```python
from build123d import *

# Parameters (mm, degrees)
BOSS_EXTRUDE1_DEPTH = 38.1
SKETCH2_R           = 17.78
CUT_EXTRUDE1_DEPTH  = 142.514046179


with BuildPart() as part:
    # Sketch1 → Boss-Extrude1 (new body, symmetric)
    with BuildSketch(Plane.XY):
        with BuildLine():
            Line((0, 0), (-177.8, 0))
            Line((-177.8, 0), (-454.042613489, -128.814046179))
            Line((-454.042613489, -128.814046179), (-459.409865413, -117.303937283))
            Line((-459.409865413, -117.303937283), (-183.167251924, 11.510108895))
            ThreePointArc((-183.167251924, 11.510108895), (-180.548783097, 12.39895929), (-177.8, 12.7))
            Line((-177.8, 12.7), (0, 12.7))
            Line((0, 12.7), (0, 0))
        make_face()
    extrude(amount=BOSS_EXTRUDE1_DEPTH, both=True)

    # Sketch2 → Cut-Extrude1 (cut, through all)
    with BuildSketch(Plane(origin=(0, 12.7, 0), x_dir=(1, 0, 0), z_dir=(0, 1, 0))):
        with Locations((-38.1, 0)):
            Circle(SKETCH2_R)
    extrude(amount=-CUT_EXTRUDE1_DEPTH, mode=Mode.SUBTRACT)


solid = part.part
```
CAD build for the part. Positions are in the model's coordinates, mm. A direction names the side the tool comes from. Round coordinates to 2 decimals unless told otherwise and drop trailing zeros. Order: outer loops, then holes, each group sorted by start corner. A loop starts at its lowest first (then second) coordinate and runs counter-clockwise, first axis right, second up. Notation, with made-up numbers: (67.25, 3.5) -> (123.25, 3.5) arc R29 ccw to (123.25, 35.5) -> close; hole circle Ø4 at (48, 25). An arc over 180 degrees is marked (long way). Write item = value, one per line.
(1) Cut at C-C (z = 26). Write the cut outline in (x, y), plus the area to 3 significant figures.
Answers follow:
outline = (-459.41, -117.3) -> (-454.04, -128.81) -> (-177.8, 0) -> (0, 0) -> (0, 12.7) -> (-177.8, 12.7) arc R12.7 ccw to (-183.17, 11.51) -> close
area = 6,160 mm²
(2) Cut at A-A (x = -38.1). Write the cut outline in (y, z).
Answers follow:
outline = (0, -38.1) -> (12.7, -38.1) -> (12.7, -17.78) -> (0, -17.78) -> close; (0, 17.78) -> (12.7, 17.78) -> (12.7, 38.1) -> (0, 38.1) -> close
(3) 3-axis set-ups, long thin cutter, end or side, ignore diameter. For faces 1 (the flat face through (-246, -26, -38.1)), 2 (the flat face through (-88, 0, 1)): which of +Z, -Z, +X, -X, +Y, -Y reach the whole face in a straight line?
Answers follow:
face_1 = -Z, +X, -X, +Y, -Y
face_2 = +Z, -Z, +X, -Y
(4) Drill centre lines: L1, parallel to Z at x = -38, y = 8; L2, parallel to Y at x = -89, z = -26; L3, parallel to X at y = 3, z = 0. Where is each one in solid material? Low to high.
Answers follow:
L1 = -38.1 to -17.78, 17.78 to 38.1
L2 = 0 to 12.7
L3 = -201.42 to -55.88, -20.32 to 0
(5) Flat gauge pins, fed straight in: P1, Ø1, axis at y = -104.5, z = -28.5, coming from the +X side; P2, Ø3, axis at x = -233, z = 9, coming from the -Y side; P3, Ø1, axis at x = -296, z = -6.5, coming from the -Y side. Where does each tip first touch, or does it go through?
Answers follow:
P1 = -400.83
P2 = -26.44
P3 = -55.35
(6) Cut at D-D (x = -136). Write the cut outline in (y, z).
Answers follow:
outline = (0, -38.1) -> (12.7, -38.1) -> (12.7, 38.1) -> (0, 38.1) -> close
(7) Pull direction X, two halves, no side cores. Call faces 3 (the flat face through (-90, 12.7, 1)), 4 (the cylindrical face through (-21.676, 6.439, 6.81)), 5 (the flat face through (0, 6, 1)): +X half, -X half, draft (parallel to the pull), parting line (faces both ways), or undercut.
Answers follow:
face_3 = draft
face_4 = undercut
face_5 = +X half
(8) Cut at B-B (z = 0). Write the cut outline in (x, y), plus the area to 3 significant figures.
Answers follow:
outline = (-459.41, -117.3) -> (-454.04, -128.81) -> (-177.8, 0) -> (-55.88, 0) -> (-55.88, 12.7) -> (-177.8, 12.7) arc R12.7 ccw to (-183.17, 11.51) -> close; (-20.32, 0) -> (0, 0) -> (0, 12.7) -> (-20.32, 12.7) -> close
area = 5,710 mm²
